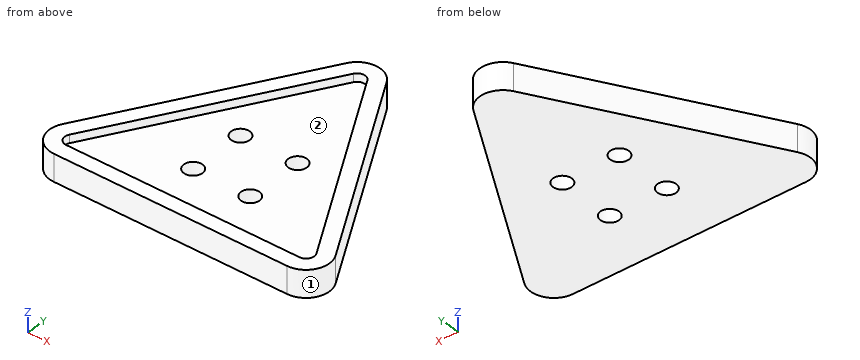
from build123d import *

# Parameters (mm, degrees)
SKETCH1_R           = 1.6
BOSS_EXTRUDE1_DEPTH = 4.6
CUT_EXTRUDE3_DEPTH  = 1.4


with BuildPart() as part:
    # Sketch1 → Boss-Extrude1 (new body)
    with BuildSketch(Plane.XY):
        with BuildLine():
            Line((-3.464101615, 25.333333333), (-23.671361037, -9.666666667))
            ThreePointArc((-23.671361037, -9.666666667), (-23.671361037, -13.666666667), (-20.207259422, -15.666666667))
            Line((-20.207259422, -15.666666667), (20.207259422, -15.666666667))
            ThreePointArc((20.207259422, -15.666666667), (23.671361037, -13.666666667), (23.671361037, -9.666666667))
            Line((23.671361037, -9.666666667), (3.464101615, 25.333333333))
            ThreePointArc((3.464101615, 25.333333333), (0, 27.333333333), (-3.464101615, 25.333333333))
        make_face()
        with Locations((-4.949747468, 4.949747468)):
            Circle(SKETCH1_R, mode=Mode.SUBTRACT)
        with Locations((4.949747468, 4.949747468)):
            Circle(SKETCH1_R, mode=Mode.SUBTRACT)
        with Locations((4.949747468, -4.949747468)):
            Circle(SKETCH1_R, mode=Mode.SUBTRACT)
        with Locations((-4.949747468, -4.949747468)):
            Circle(SKETCH1_R, mode=Mode.SUBTRACT)
    extrude(amount=BOSS_EXTRUDE1_DEPTH)

    # Sketch4 → Cut-Extrude3 (cut)
    with BuildSketch(Plane.XY.offset(4.6)):
        with BuildLine():
            Line((-20.207259422, -13.066666667), (20.207259422, -13.066666667))
            ThreePointArc((20.207259422, -13.066666667), (21.419694987, -12.366666667), (21.419694987, -10.966666667))
            Line((21.419694987, -10.966666667), (1.212435565, 24.033333333))
            ThreePointArc((1.212435565, 24.033333333), (0, 24.733333333), (-1.212435565, 24.033333333))
            Line((-1.212435565, 24.033333333), (-21.419694987, -10.966666667))
            ThreePointArc((-21.419694987, -10.966666667), (-21.419694987, -12.366666667), (-20.207259422, -13.066666667))
        make_face()
    extrude(amount=-CUT_EXTRUDE3_DEPTH, mode=Mode.SUBTRACT)


solid = part.part
For this review, take the finished solid that the model builds, in its own axes (mm). Face numbers are marked on the shaded views. A direction names the side the tool comes from. Round coordinates to 2 decimals unless told otherwise and drop trailing zeros. Loops run counter-clockwise (first coordinate to the right, second up) from the corner with the lowest first, then second, coordinate; pieces in that order, holes last. Notation, with made-up numbers: (18.25, 21.5) - (23.25, 21.5) arc R17 cw to (23.25, 47.5) - close; hole circle Ø5 at (19.25, 43). An arc over 180 degrees is marked (long way). One line per question, with ' | ' between items.
Q1. Tool access review of the marked faces 1 and 2: name each direction out of +Z, -Z, +X, -X, +Y, -Y from which nothing blocks a thin tool from reaching the whole face with its end or side.
Taken from the geometry:
face 1: +Z, -Z, +X | face 2: +Z
Q2. Take a section at A-A (x = 0). Give the boundary of the cut face in (y, z), and give its area (3 significant figures).
Taken from the geometry:
outline: (-15.67, 0) - (27.33, 0) - (27.33, 4.6) - (24.73, 4.6) - (24.73, 3.2) - (-13.07, 3.2) - (-13.07, 4.6) - (-15.67, 4.6) - close | area: 145 mm²
Q3. For line 1 along X through (y, z) = (3.5, 1.45); line 2 along Z through (x, y) = (3, 0); line 3 along X through (y, z) = (14.5, 3.65), list the stretches that pass through material, from the lowest coordinate up. Write a range as [from, to].
Taken from the geometry:
line 1: x = [-16.07, -5.63], [-4.27, 4.27], [5.63, 16.07] | line 2: z = [0, 3.2] | line 3: x = [-9.72, -6.72], [6.72, 9.72]
Q4. Take a section at B-B (x = 5). Give the boundary of the cut face in (y, z).
Taken from the geometry:
outline: (-15.67, 0) - (-6.55, 0) - (-6.55, 3.2) - (-13.07, 3.2) - (-13.07, 4.6) - (-15.67, 4.6) - close; (-3.35, 0) - (3.35, 0) - (3.35, 3.2) - (-3.35, 3.2) - close; (6.55, 0) - (22.67, 0) - (22.67, 4.6) - (17.47, 4.6) - (17.47, 3.2) - (6.55, 3.2) - close
Q5. Take a section at C-C (y = -0.5). Give the boundary of the cut face in (x, z).
Taken from the geometry:
outline: (-18.38, 0) - (18.38, 0) - (18.38, 4.6) - (15.38, 4.6) - (15.38, 3.2) - (-15.38, 3.2) - (-15.38, 4.6) - (-18.38, 4.6) - close
Q6. For pin 1 (1 mm diameter, centred on y = 19.5, z = 2.5, fed in from +X); pin 2 (1.1 mm diameter, centred on x = 2.5, z = 3.5, fed in from +Y); pin 3 (4 mm diameter, centred on x = 5.5, y = 9, fed in from +Z), all flat-tipped, find the tip position at first contact; note any pin that passes through.
Taken from the geometry:
pin 1: stops at x = 7.12 | pin 2: stops at y = 26.83 | pin 3: stops at z = 3.2
Q7. Take a section at D-D (z = 1.8). Give the boundary of the cut face in (x, y), and give its area (3 significant figures).
Taken from the geometry:
outline: (-23.67, -9.67) arc R4 ccw to (-20.21, -15.67) - (20.21, -15.67) arc R4 ccw to (23.67, -9.67) - (3.46, 25.33) arc R4 ccw to (-3.46, 25.33) - close; hole circle Ø3.2 at (-4.95, -4.95); hole circle Ø3.2 at (-4.95, 4.95); hole circle Ø3.2 at (4.95, -4.95); hole circle Ø3.2 at (4.95, 4.95) | area: 1,210 mm²
